from build123d import *

# Parameters (mm, degrees)
F0_W      = 342.9
F0_H      = 177.8
F0_W_2    = 228.6
F0_H_2    = 215.9
F1_DEPTH  = 25.4
F2_W      = 304.8
F2_H      = 12.7
F3_DEPTH  = 12.7
F4_W      = 304.8
F4_H      = 12.7
F5_DEPTH  = 12.7
F6_R      = 12.7
F7_DEPTH  = 25.4
F9_DEPTH  = 12.7
F10_W     = 190.5
F10_H     = 19.05
F11_DEPTH = 12.7
F12_W     = 292.1
F12_H     = 12.7
F13_DEPTH = 12.7


with BuildPart() as f1:
    # F0 (on Front) → F1 (new body)
    with BuildSketch(Plane.XZ):
        with Locations((171.45, 88.9)):
            Rectangle(F0_W, F0_H)
        Polygon((0, 241.3), (0, 177.8), (342.9, 177.8), (342.9, 241.3), (285.75, 241.3), (57.15, 241.3), align=None)
        with Locations((171.45, 349.25)):
            Rectangle(F0_W_2, F0_H_2)
    extrude(amount=F1_DEPTH)

    # F2 (on face) → F3 (cut)
    with BuildSketch(Plane.XZ.offset(25.4)):
        with Locations((177.8, 12.7)):
            Rectangle(F2_W, F2_H)
    extrude(amount=-F3_DEPTH, mode=Mode.SUBTRACT)

    # F4 (on face) → F5 (cut)
    with BuildSketch(Plane.XZ.offset(25.4)):
        with Locations((177.8, -12.7)):
            Rectangle(F4_W, F4_H)
    extrude(amount=-F5_DEPTH, mode=Mode.SUBTRACT)

    # F6 (on face) → F7 (cut)
    with BuildSketch(Plane(origin=(0, 0, 0), x_dir=(-1, 0, 0), z_dir=(0, 1, 0))):
        with Locations((-63.5, 38.1)):
            Circle(F6_R)
    extrude(amount=-F7_DEPTH, mode=Mode.SUBTRACT)

    # F8 (on face) → F9 (cut)
    with BuildSketch(Plane.XZ.offset(25.4)):
        Polygon((323.85, 44.45), (330.2, 44.45), (336.55, 44.45), (336.55, 133.35), (323.85, 133.35), align=None)
    extrude(amount=-F9_DEPTH, mode=Mode.SUBTRACT)

    # F10 (on face) → F11 (cut)
    with BuildSketch(Plane.XZ.offset(25.4)):
        with Locations((171.45, 447.675)):
            Rectangle(F10_W, F10_H)
        Polygon((76.2, 438.15), (76.2, 457.2), (57.15, 457.2), (57.15, 241.3), (76.2, 241.3), align=None)
        Polygon((285.75, 241.3), (285.75, 457.2), (266.7, 457.2), (266.7, 438.15), (266.7, 241.3), align=None)
    extrude(amount=-F11_DEPTH, mode=Mode.SUBTRACT)

    # F12 (on face) → F13 (cut)
    with BuildSketch(Plane.XZ.offset(25.4)):
        with Locations((171.45, 209.55)):
            Rectangle(F12_W, F12_H)
        with Locations((171.45, 184.15)):
            Rectangle(F12_W, F12_H)
    extrude(amount=-F13_DEPTH, mode=Mode.SUBTRACT)


solid = f1.part
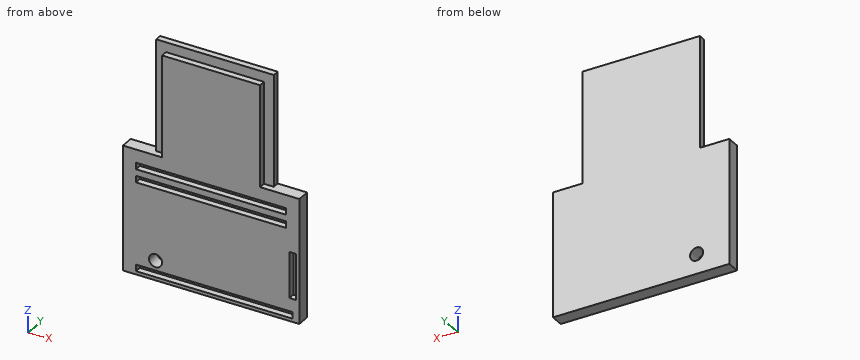
Check sheet for the modelled part. Datum: model origin and axes. Units: mm. Round coordinates to 2 decimals unless told otherwise and drop trailing zeros. Order: outer loops, then holes, each group sorted by start corner. A loop starts at its lowest first (then second) coordinate and runs counter-clockwise, first axis right, second up.
(1) Scan lines: probe 1 along Z at (x, y) = (220, -16.5); probe 2 along Z at (x, y) = (63.5, -16); probe 3 along Z at (x, y) = (63.5, -9.75). Record each from-to range of solid material in increasing order.
(2) Cross-section at C-C, the plane y = -19. Enter the section's corners in (x, z), and give its area (3 significant figures).
(3) Cross-section at D-D, the plane z = 95.5. Enter the section's corners in (x, y).
(4) Cross-section at A-A, the plane x = 63.5. Enter the section's corners in (y, z).
(5) Cross-section at B-B, the plane z = 38.1. Enter the section's corners in (x, y).
(6) Go/stop test with flat-tipped pins: P1, Ø4, axis at y = -7, z = 364.5, coming from the +X side; P2, Ø7.5, axis at x = 39, y = -9, coming from the +Z side; P3, Ø4, axis at y = -21.5, z = 304.5, coming from the +X side; P4, Ø1.5, axis at x = 235.5, y = -12.5, coming from the -Z side. Record where each tip stops, or that it passes through.
Check sheet entries:
1. probe 1: z = 0 to 6.35, 19.05 to 177.8, 190.5 to 203.2, 215.9 to 438.15
1. probe 2: z = 0 to 6.35, 19.05 to 25.4, 50.8 to 177.8, 190.5 to 203.2, 215.9 to 241.3
1. probe 3: z = 0 to 25.4, 50.8 to 457.2
2. outline: (0, 0) - (342.9, 0) - (342.9, 241.3) - (266.7, 241.3) - (266.7, 438.15) - (76.2, 438.15) - (76.2, 241.3) - (0, 241.3) - close; hole (25.4, 6.35) - (330.2, 6.35) - (330.2, 19.05) - (25.4, 19.05) - close; hole (25.4, 177.8) - (317.5, 177.8) - (317.5, 190.5) - (25.4, 190.5) - close; hole (25.4, 203.2) - (317.5, 203.2) - (317.5, 215.9) - (25.4, 215.9) - close; hole circle Ø25.4 at (63.5, 38.1); hole (323.85, 44.45) - (336.55, 44.45) - (336.55, 133.35) - (323.85, 133.35) - close
2. area: 107,000 mm2
3. outline: (0, -25.4) - (323.85, -25.4) - (323.85, -12.7) - (336.55, -12.7) - (336.55, -25.4) - (342.9, -25.4) - (342.9, 0) - (0, 0) - close
4. outline: (-25.4, 0) - (0, 0) - (0, 25.4) - (-25.4, 25.4) - (-25.4, 19.05) - (-12.7, 19.05) - (-12.7, 6.35) - (-25.4, 6.35) - close; (-25.4, 50.8) - (0, 50.8) - (0, 457.2) - (-12.7, 457.2) - (-12.7, 241.3) - (-25.4, 241.3) - (-25.4, 215.9) - (-12.7, 215.9) - (-12.7, 203.2) - (-25.4, 203.2) - (-25.4, 190.5) - (-12.7, 190.5) - (-12.7, 177.8) - (-25.4, 177.8) - close
5. outline: (0, -25.4) - (50.8, -25.4) - (50.8, 0) - (0, 0) - close; (76.2, -25.4) - (342.9, -25.4) - (342.9, 0) - (76.2, 0) - close
6. P1: stops at x = 285.75
6. P2: stops at z = 241.3
6. P3: stops at x = 266.7
6. P4: stops at z = 0
